Verification items for the finished model (mm, model axes). Face numbers are marked on the shaded views. A direction names the side the tool comes from. Round coordinates to 2 decimals unless told otherwise and drop trailing zeros. Order: outer loops, then holes, each group sorted by start corner. A loop starts at its lowest first (then second) coordinate and runs counter-clockwise, first axis right, second up. Notation, with made-up numbers: (70, 24) -> (128, 24) arc R12 ccw to (128, 34) -> close; hole circle Ø2 at (3.5, 46.5). An arc over 180 degrees is marked (long way). Put each result on its own line as item: value.
from build123d import *

# Parameters (mm, degrees)
SKETCH2_R          = 1.25
CUT_EXTRUDE1_DEPTH = 10
CIRPATTERN1_COUNT  = 2
CIRPATTERN1_ANGLE  = 270


with BuildPart() as part:
    # Sketch1 → Revolve1 (revolve)
    with BuildSketch(Plane.XY, mode=Mode.PRIVATE) as revolve1_sk:
        Polygon((0, 0), (25, 0), (25, 6), (12.5, 6), (12.5, 7.5), (0, 7.5), align=None)
    revolve(revolve1_sk.sketch.rotate(Axis((0, 10, 0), (1, 0, 0)), 270), axis=Axis((0, 10, 0), (1, 0, 0)))

    # Sketch2 → Cut-Extrude1 (cut)
    with BuildSketch(Plane.XY):
        with Locations((22.5, 10)):
            Circle(SKETCH2_R)
        with Locations((2.5, 10)):
            Circle(SKETCH2_R)
    cut_extrude1 = extrude(amount=-CUT_EXTRUDE1_DEPTH, mode=Mode.SUBTRACT)

    # CirPattern1: Cut-Extrude1 ×2 about axis
    cirpattern1_axis = Axis((0, 10, 0), (1, 0, 0))
    for i in range(1, CIRPATTERN1_COUNT):
        add(cut_extrude1.rotate(cirpattern1_axis, i * CIRPATTERN1_ANGLE / (CIRPATTERN1_COUNT - 1)), mode=Mode.SUBTRACT)


solid = part.part
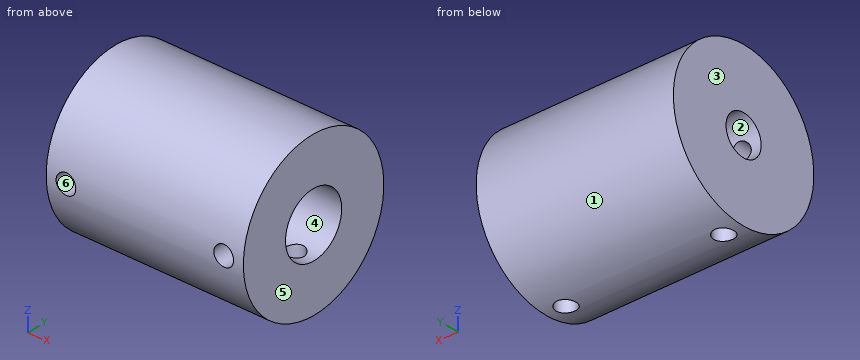
Item 1: Section check C-C on x = 13. Record the boundary of the cut face in (y, z).
Check sheet entries:
outline: circle Ø20 at (10, 0); hole circle Ø8 at (10, 0)
Item 2: Material ranges on L1, parallel to X at y = 10, z = -7.5; L2, parallel to Y at x = 22.5, z = -8; L3, parallel to Y at x = 19, z = -2.25, recorded low to high. Write a range as [from, to].
Check sheet entries:
L1: x = [0, 1.25], [3.75, 21.25], [23.75, 25]
L2: y = [4, 8.75], [11.25, 16]
L3: y = [0.26, 6.69], [13.31, 19.74]
Item 3: Section check D-D on y = 7. Record the boundary of the cut face in (x, z).
Check sheet entries:
outline: (0, -9.54) -> (25, -9.54) -> (25, -2.65) -> (12.5, -2.65) -> (12.5, 2.65) -> (25, 2.65) -> (25, 9.54) -> (0, 9.54) -> close; hole circle Ø2.5 at (2.5, 0)
Item 4: Tool access check on the marked faces 4, 5 and 6. Record the directions out of +Z, -Z, +X, -X, +Y, -Y that give a thin tool (end or side, any length) a straight path to the whole face; none if there is none.
Check sheet entries:
face 4: +X
face 5: +Z, -Z, +X, +Y, -Y
face 6: -Y
Item 5: Gauge pin test, flat ends, axial feed: pin 1 Ø12 at (x, z) = (17.5, -6.5) entering from -Y; pin 2 Ø6 at (x, z) = (5, 7) entering from +Y; pin 3 Ø4 at (x, z) = (17.5, -7.5) entering from -Y; pin 4 Ø2.5 at (y, z) = (10, -1) entering from +X. Record the tip position at first contact, or that the pin passes through.
Check sheet entries:
pin 1: stops at y = 0.01
pin 2: stops at y = 19.17
pin 3: stops at y = 1.65
pin 4: passes through
Item 6: Release check for a two-part mould opening along Y. For the marked faces 1, 2 and 3 record: +Y half, -Y half, draft (parallel to the pull), parting line (faces both ways), or undercut.
Check sheet entries:
face 1: parting line
face 2: undercut
face 3: draft
Item 7: Section check A-A on z = 0. Record the boundary of the cut face in (x, y), then the cut area to 3 significant figures.
Check sheet entries:
outline: (0, 0) -> (1.25, 0) -> (1.25, 7.5) -> (0, 7.5) -> close; (0, 12.5) -> (12.5, 12.5) -> (12.5, 14) -> (25, 14) -> (25, 20) -> (0, 20) -> close; (3.75, 0) -> (21.25, 0) -> (21.25, 6) -> (12.5, 6) -> (12.5, 7.5) -> (3.75, 7.5) -> close; (23.75, 0) -> (25, 0) -> (25, 6) -> (23.75, 6) -> close
area: 304 mm^2
Item 8: Section check B-B on y = 10. Record the boundary of the cut face in (x, z).
Check sheet entries:
outline: (0, -10) -> (1.25, -10) -> (1.25, -2.5) -> (0, -2.5) -> close; (0, 2.5) -> (12.5, 2.5) -> (12.5, 4) -> (25, 4) -> (25, 10) -> (0, 10) -> close; (3.75, -10) -> (21.25, -10) -> (21.25, -4) -> (12.5, -4) -> (12.5, -2.5) -> (3.75, -2.5) -> close; (23.75, -10) -> (25, -10) -> (25, -4) -> (23.75, -4) -> close
